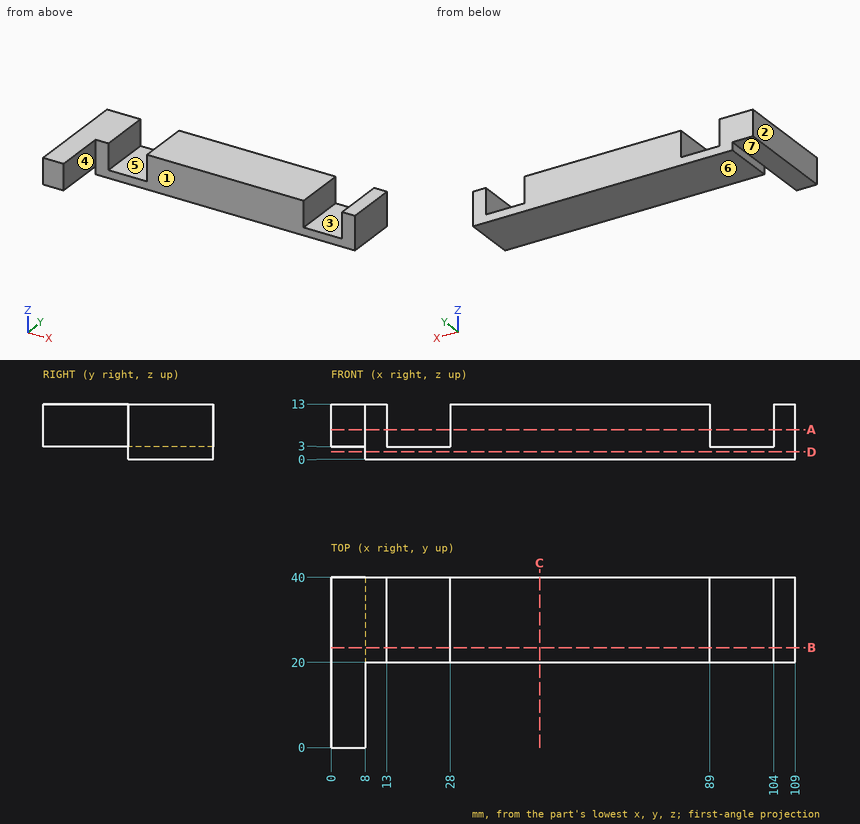
Print and shaded views of the part. All mm, measured from the part's lowest x, y and z. A direction names the side the tool comes from. Round coordinates to 2 decimals unless told otherwise and drop trailing zeros. Write each loop counter-clockwise with the first axis right and the second up, starting at its lowest first coordinate (ties: lowest second). Pieces come first, ordered by that corner, then holes.
(1) Slice it at D-D, the plane z = 1.75. Write the cut outline in (x, y), and give its area (3 significant figures).
(2) 3-axis set-ups, long thin cutter, end or side, ignore diameter. For the marked faces 5, 6 and 7: which of +Z, -Z, +X, -X, +Y, -Y reach the whole face in a straight line?
(3) Slice it at C-C, the plane x = 49. Write the cut outline in (y, z), and give its area (3 significant figures).
(4) Slice it at B-B, the plane y = 23.5. Write the cut outline in (x, z).
(5) Probe line 1 along X through (y, z) = (32, 6.5); line 2 along Y through (x, z) = (53, 5.25); line 3 along Z through (x, y) = (92, 32). List the from-to ranges inside material, lowest first.
(6) Drop flat-ended pins along their axis: P1, Ø4.5, axis at x = 21, y = 29, coming from the +Z side; P2, Ø2, axis at x = 89.5, z = 3.5, coming from the -Y side; P3, Ø1, axis at y = 6, z = 3, coming from the +X side; P4, Ø1.5, axis at x = 27, z = 9, coming from the -Y side. Give the stop position or say it passes through.
(7) Mould opens along X. For the marked faces 1, 2, 3 and 4 say: pulls with the +X half, pulls with the -X half, needs draft (parallel to the pull), parting line crosses it, or undercut.
(8) Slice it at A-A, the plane z = 7. Write the cut outline in (x, y).
From the geometry:
1. outline: (8, 20) - (109, 20) - (109, 40) - (8, 40) - close
1. area: 2,020 mm2
2. face 5: +Z, +Y, -Y
2. face 6: -Z, +X, -X, +Y, -Y
2. face 7: -Z, -X, +Y, -Y
3. outline: (20, 0) - (40, 0) - (40, 13) - (20, 13) - close
3. area: 260 mm2
4. outline: (0, 3) - (8, 3) - (8, 0) - (109, 0) - (109, 13) - (104, 13) - (104, 3) - (89, 3) - (89, 13) - (28, 13) - (28, 3) - (13, 3) - (13, 13) - (0, 13) - close
5. line 1: x = 0 to 13, 28 to 89, 104 to 109
5. line 2: y = 20 to 40
5. line 3: z = 0 to 3
6. P1: stops at z = 3
6. P2: stops at y = 20
6. P3: stops at x = 8
6. P4: passes through
7. face 1: needs draft
7. face 2: pulls with the -X half
7. face 3: undercut
7. face 4: pulls with the +X half
8. outline: (0, 0) - (8, 0) - (8, 20) - (13, 20) - (13, 40) - (0, 40) - close; (28, 20) - (89, 20) - (89, 40) - (28, 40) - close; (104, 20) - (109, 20) - (109, 40) - (104, 40) - close
